Model file for the job. Use its own axes, mm. A direction names the side the tool comes from. Coordinates: 2 decimals unless noted, no trailing zeros. Order: outer loops, then holes, each group sorted by start corner. A loop starts at its lowest first (then second) coordinate and runs counter-clockwise, first axis right, second up. Notation, with made-up numbers: (-29, 41) -> (7, 41) arc R14 cw to (7, 56) -> close; hole circle Ø2 at (69, 85). An arc over 180 degrees is marked (long way). Write item = value, one per line. Start each with the question number.
Q1. Cut at A-A, the plane z = 9. List the corners of the cut face in (x, y) (3 decimals), plus the area to 3 significant figures.
Q2. Mould opens along X. For faces 1 (the face through (55.377, 8.593, 8.944)), 2 (the face through (55, 9, 5)), 3 (the face through (0, 14, 5)) say: +X half, -X half, draft (parallel to the pull), parting line (faces both ways), or undercut.
Q3. Cut at B-B, the plane x = -52. List the corners of the cut face in (y, z), plus the area to 3 significant figures.
Q4. Flat gauge pins, fed straight in: pin 1 (4 mm diameter, centred on x = 57, y = 7, fed in from +Z); pin 2 (2.5 mm diameter, centred on x = 3.5, z = 8, fed in from +Y); pin 3 (2.5 mm diameter, centred on x = 56.5, y = 7.5, fed in from -Z); pin 4 (12 mm diameter, centred on x = -3, y = 5.5, fed in from +Z). Where does each tip first touch, or does it go through?
Q5. Wall check: line 1 (Y direction, x = 57.5, z = 9) (3 decimals); line 2 (X direction, y = 8.25, z = 7.25); line 3 (X direction, y = 13.75, z = 4). Give the ranges that are in metal, low to high. Write a range as from..to.
Q6. 3-axis set-ups, long thin cutter, end or side, ignore diameter. For faces 4 (the face through (-71.48, 4.85, 4.24)), 5 (the face through (5, 17, 9)), 6 (the face through (55, 3.5, 9)), 7 (the face through (55, 9, 13)): which of +Z, -Z, +X, -X, +Y, -Y reach the whole face in a straight line?
from build123d import *

# Parameters (mm, degrees)
BASE_DEPTH       = 18
SKETCH2_R        = 2.125
MOUNT_DEPTH      = 4
MOUNT_DEPTH_BACK = 4
SKETCH3_R        = 6
TUBE_DEPTH       = 145
FILLET1_R        = 1


with BuildPart() as part:
    # Sketch1 → Base (new body)
    with BuildSketch(Plane.XY):
        Polygon((0, 0), (53, 0), (53, 20), (9.30875576, 20), (9.30875576, 17), (0, 17), align=None)
    extrude(amount=BASE_DEPTH)

    # Sketch2 → Mount (add, two sides)
    with BuildSketch(Plane.XY.offset(9)) as mount_sk:
        with BuildLine():
            Line((53, 13.5), (57.75, 13.5))
            ThreePointArc((57.75, 13.5), (60.75520382, 12.25520382), (62, 9.25))
            Line((62, 9.25), (62, 7.75))
            ThreePointArc((62, 7.75), (60.75520382, 4.74479618), (57.75, 3.5))
            Line((57.75, 3.5), (53, 3.5))
            Line((53, 3.5), (53, 13.5))
        make_face()
        with Locations((57.5, 8.5)):
            Circle(SKETCH2_R, mode=Mode.SUBTRACT)
    extrude(amount=MOUNT_DEPTH)
    extrude(mount_sk.sketch, amount=-MOUNT_DEPTH_BACK)

    # Sketch3 → Tube (add)
    with BuildSketch(Plane.ZY):
        with Locations((9, 8.5)):
            Circle(SKETCH3_R)
    extrude(amount=TUBE_DEPTH)

    # Fillet1
    fillet1_edges = [part.edges().sort_by_distance(p)[0] for p in [
        (53, 10, 18),
        (0, 17, 9),
        (9.30875576, 20, 9),
        (53, 20, 9),
        (53, 0, 9),
        (0, 0, 9),
        (31.15437788, 20, 18),
        (9.30875576, 18.5, 18),
        (4.65437788, 17, 18),
        (55.375, 13.5, 5),
        (60.75520382, 12.25520382, 5),
        (62, 8.5, 5),
        (60.75520382, 4.74479618, 5),
        (55.375, 3.5, 5),
        (55.375, 3.5, 13),
        (60.75520382, 4.74479618, 13),
        (62, 8.5, 13),
        (60.75520382, 12.25520382, 13),
        (55.375, 13.5, 13),
        (0, 8.5, 18),
        (4.65437788, 17, 0),
        (9.30875576, 18.5, 0),
        (31.15437788, 20, 0),
        (26.5, 0, 18),
        (53, 10, 0),
        (26.5, 0, 0),
        (0, 8.5, 0),
    ]]
    fillet(fillet1_edges, radius=FILLET1_R)


solid = part.part
Here are the results:
q1.outline = (-145, 2.5) -> (0, 2.5) -> (0, 1) arc R1 ccw to (1, 0) -> (52, 0) arc R1 ccw to (53, 1) -> (53, 3.5) -> (57.75, 3.5) arc R4.25 ccw to (62, 7.75) -> (62, 9.25) arc R4.25 ccw to (57.75, 13.5) -> (53, 13.5) -> (53, 19) arc R1 ccw to (52, 20) -> (10.309, 20) arc R1 ccw to (9.309, 19) -> (9.309, 17) -> (1, 17) arc R1 ccw to (0, 16) -> (0, 14.5) -> (-145, 14.5) -> close; hole circle Ø4.25 at (57.5, 8.5)
q1.area = 2,840 mm²
q2.face_1 = undercut
q2.face_2 = draft
q2.face_3 = -X half
q3.outline = circle Ø12 at (8.5, 9)
q3.area = 113 mm²
q4.pin_1 = 13
q4.pin_2 = 17
q4.pin_3 = 5
q4.pin_4 = 18
q5.line_1 = 3.5..6.375, 10.625..13.5
q5.line_2 = -145..55.39, 59.61..62
q5.line_3 = 0..53
q6.face_4 = -X
q6.face_5 = +Z, -Z, -X, +Y
q6.face_6 = +Z, -Z, +X, -Y
q6.face_7 = +Z, +X, +Y, -Y
